For this review, take the finished solid that the model builds, in its own axes (mm). A direction names the side the tool comes from. Give positions to 0.01 mm unless a question says otherwise; leave off trailing zeros. Write each loop counter-clockwise with the first axis right and the second up, starting at its lowest first coordinate (ties: lowest second). Pieces come first, ordered by that corner, then holes. Notation, with made-up numbers: M 6,28.5 L 56,28.5 A34 ccw 56,66.5 Z; hole C 85,66.5 d8. An arc over 180 degrees is marked long. Write item = value, one per line.
Autodesk Inventor part; units mm, degrees
ref_plane "YZ Plane" through (0, 0, 0) normal (1, 0, 0) x (0, 1, 0)
ref_plane "XZ Plane" through (0, 0, 0) normal (0, 1, 0) x (-1, 0, 0)
ref_plane "XY Plane" through (0, 0, 0) normal (0, 0, 1) x (1, 0, 0)
sketch "Sketch1" plane through (0, 0, 0) normal (0, 0, 1) x (1, 0, 0)
  line L0 (-33.02, 0) -> (-33.02, 114.3)
  line L1 (-33.02, 114.3) -> (0, 114.3)
  line L2 (0, 114.3) -> (0, 0)
  line L3 (-33.02, 0) -> (-26.67, 0)
  line L4 (-26.67, 0) -> (-26.67, 107.95)
  line L5 (-33.02, 114.3) -> (-33.02, 107.95)
  line L6 (-26.67, 107.95) -> (-6.35, 107.95)
  line L7 (0, 114.3) -> (-6.35, 114.3)
  line L8 (-6.35, 107.95) -> (-6.35, 0)
  line L9 (0, 0) -> (-6.35, 0)
  line L10 (-26.67, 0) -> (-33.02, 0)
  dimension "d0" = 33.02
  dimension "d1" = 114.3
  dimension "d2" = 6.35
  dimension "d3" = 6.35
  dimension "d4" = 6.35
  dimension "d11" = 114.3
extrude "Extrusion1" add sketch "Sketch1" along normal blind 25.4
sketch "Sketch2" plane through (0, 0, 0) normal (1, 0, 0) x (0, 0, -1)
  line L0 (0, 0) -> (-25.4, 0)
  line L1 (0, 114.3) -> (-25.4, 114.3)
  line L2 (-12.7, 0) -> (-12.7, 19.05)
  circle A0 centre (-12.7, 19.05) radius 6.35
  dimension "d7" = 19.05
  dimension "d8" = 12.7
extrude "Extrusion2" cut sketch "Sketch2" against normal blind 254
sketch "Sketch3" plane through (-33.02, 114.3, 0) normal (0, 1, 0) x (1, 0, 0)
  circle A0 centre (16.51, -12.7) radius 6.35
  dimension "d12" = 12.7
extrude "Extrusion3" add sketch "Sketch3" along normal blind 19.05
properties part number "wheel support"
1. For line 1 along Y through (x, z) = (-28.75, 12.7); line 2 along X through (y, z) = (97, 13.25); line 3 along Z through (x, y) = (-2.5, 19.05), list the stretches that pass through material, from the lowest coordinate up. Write a range as from..to.
Responses:
line_1 = 0..12.7, 25.4..114.3
line_2 = -33.02..-26.67, -6.35..0
line_3 = 0..6.35, 19.05..25.4
2. The part is to be moulded in two halves that separate along X. For faces 4 (the face through (0, 58, 13)), 5 (the face through (-17, 107.95, 13)), 6 (the face through (-6, 58, 25.4)), say which applies: +X half, -X half, draft (parallel to the pull), parting line (faces both ways), or undercut.
Responses:
face_4 = +X half
face_5 = undercut
face_6 = draft
3. We need section A-A, the plane z = 12.7. Write out the cut boundary in (x, y).
Responses:
outline = M -33.02,0 L -26.67,0 L -26.67,12.7 L -33.02,12.7 Z; M -33.02,25.4 L -26.67,25.4 L -26.67,107.95 L -6.35,107.95 L -6.35,25.4 L 0,25.4 L 0,114.3 L -10.16,114.3 L -10.16,133.35 L -22.86,133.35 L -22.86,114.3 L -33.02,114.3 Z; M -6.35,0 L 0,0 L 0,12.7 L -6.35,12.7 Z
4. Machinability: for faces 1 (the face through (-13.096, 123.692, 18.054)), 2 (the face through (-33.02, 56, 13)), 3 (the face through (-6.35, 55, 13)), which of the approach directions +Z, -Z, +X, -X, +Y, -Y give a long, thin tool a straight path to every point of the face, cutting with its end or side? Answer none if there is none.
Responses:
face_1 = +Y
face_2 = +Z, -Z, -X, +Y, -Y
face_3 = +Z, -Z, -Y
5. We need section C-C, the plane y = 85. Write out the cut boundary in (x, z).
Responses:
outline = M -33.02,0 L -26.67,0 L -26.67,25.4 L -33.02,25.4 Z; M -6.35,0 L 0,0 L 0,25.4 L -6.35,25.4 Z
6. We need section B-B, the plane y = 19.05. Write out the cut boundary in (x, z).
Responses:
outline = M -33.02,0 L -26.67,0 L -26.67,6.35 L -33.02,6.35 Z; M -33.02,19.05 L -26.67,19.05 L -26.67,25.4 L -33.02,25.4 Z; M -6.35,0 L 0,0 L 0,6.35 L -6.35,6.35 Z; M -6.35,19.05 L 0,19.05 L 0,25.4 L -6.35,25.4 Z
7. Insertion check: P1, Ø1, axis at x = -26, z = 21, coming from the +Y side; P2, Ø1, axis at x = -14, z = 15, coming from the -Y side. Each pin has a flat end and moves straight along its axis. Give the tip position at first contact, or say it passes through.
Responses:
P1 = 114.3
P2 = 107.95
8. We need section D-D, the plane x = -16.51. Write out the cut boundary in (y, z), then the cut area to 3 significant figures.
Responses:
outline = M 107.95,0 L 114.3,0 L 114.3,6.35 L 133.35,6.35 L 133.35,19.05 L 114.3,19.05 L 114.3,25.4 L 107.95,25.4 Z
area = 403 mm2
